from build123d import *

# Parameters (mm, degrees)
SKETCH1_R               = 2.38125
BOSS_EXTRUDE1_DEPTH     = 69.85
SKETCH7_R               = 1.984375
CUT_EXTRUDE1_DEPTH      = 3.38125
CUT_EXTRUDE1_DEPTH_BACK = 3.38125


with BuildPart() as part:
    # Sketch1 → Boss-Extrude1 (new body)
    with BuildSketch(Plane(origin=(0, 0, 0), x_dir=(1, 0, 0), z_dir=(0, 1, 0))):
        Circle(SKETCH1_R)
    extrude(amount=BOSS_EXTRUDE1_DEPTH)

    # Sketch2 → Revolve4 (revolve)
    with BuildSketch(Plane.XY):
        Polygon((0, 76.2), (0, 69.85), (0.8128, 69.85), (0.8128, 75.157753569), align=None)
    revolve(axis=Axis((0, 79.243977314, 0), (0, -1, 0)))

    # Sketch4 → Revolve5 (revolve)
    with BuildSketch(Plane(origin=(0, 0, 0), x_dir=(0, 0, -1), z_dir=(1, 0, 0))):
        Polygon((0, 0), (-0.054059899, -6.35), (0.8128, -4.848554612), (0.8128, 0), align=None)
    revolve(axis=Axis((0, 0, 0), (0, -0.999963763, 0.008513061)))

    # Sketch7 → Cut-Extrude1 (cut, two sides)
    with BuildSketch(Plane(origin=(0, 0, 0), x_dir=(0, 0, -1), z_dir=(1, 0, 0))) as cut_extrude1_sk:
        with Locations((0, 63.5)):
            Circle(SKETCH7_R)
    extrude(amount=CUT_EXTRUDE1_DEPTH, mode=Mode.SUBTRACT)
    extrude(cut_extrude1_sk.sketch, amount=-CUT_EXTRUDE1_DEPTH_BACK, mode=Mode.SUBTRACT)


solid = part.part
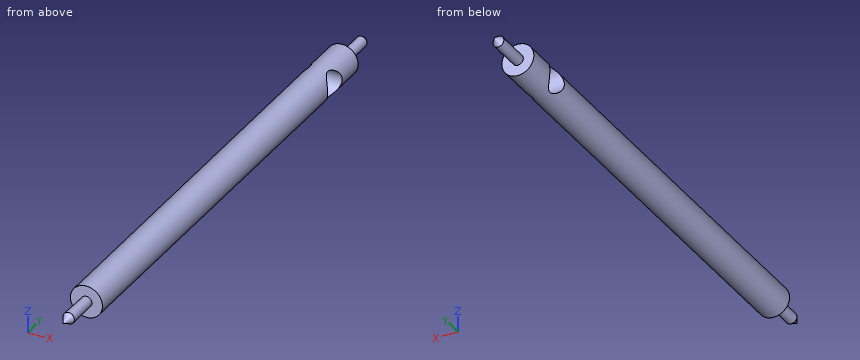
Geometry: final body of the model. Coordinates: model frame, mm. Round coordinates to 2 decimals unless told otherwise and drop trailing zeros. Loops run counter-clockwise (first coordinate to the right, second up) from the corner with the lowest first, then second, coordinate; pieces in that order, holes last. Notation, with made-up numbers: (-11.75, -28) - (46.25, -28) arc R17 ccw to (46.25, -12) - close; hole circle Ø11 at (1.5, 13.25). An arc over 180 degrees is marked (long way). Write each question's results on one line, items separated by ' | '. Start each with the question number.
1) Cut plane B-B on y = 18. Return loops of the section in (x, z).
2) Cut plane A-A on y = 63.5. Return loops of the section in (x, z), then the cut area to 3 significant figures.
3) Line query: probe 1 along Y at (x, z) = (1.6, 0); probe 2 along Z at (x, y) = (0.1, 41); probe 3 along X at (y, z) = (43, 0.25). Output: solid intervals per line, ascending. Write a range as [from, to].
4) First-contact query: P1, Ø2, axis at x = 0.5, z = -1.5, coming from the +Y side; P2, Ø2, axis at x = -1.5, y = 15.5, coming from the -Z side; P3, Ø1.5, axis at x = 1.5, z = -2, coming from the +Y side. Flat tips, straight axial feed; report the tip coordinate or a pass-through.
Verdict:
1) outline: circle Ø4.76 at (0, 0)
2) outline: (-1.32, -1.98) arc R2.38 ccw to (1.32, -1.98) - close; (-1.32, 1.98) - (1.32, 1.98) arc R2.38 ccw to start | area: 1.42 mm2
3) probe 1: y = [0, 61.52], [65.48, 69.85] | probe 2: z = [-2.38, 2.38] | probe 3: x = [-2.37, 2.37]
4) P1: stops at y = 75.45 | P2: stops at z = -2.33 | P3: stops at y = 69.85
